Source: CAD feature listing. Evaluate the final solid. Frame: model axes, mm. Give positions to 0.01 mm unless a question says otherwise; leave off trailing zeros. Write each loop counter-clockwise with the first axis right and the second up, starting at its lowest first coordinate (ties: lowest second). Pieces come first, ordered by that corner, then holes. Notation, with made-up numbers: (27, -30) -> (86, -30) arc R36 ccw to (86, 6) -> close; hole circle Ø11 at (-28, 24.25). An arc over 180 degrees is marked (long way). Answer as a JSON object with one key per item and string values. Group by question number.
Item 1: Section query A-A on x = 48. Return the cut outline in (y, z), plus the area to 3 significant figures.
Item 2: Section query D-D on y = -6. Return the cut outline in (x, z).
Item 3: Ray query, probe 1 along Y at (x, z) = (83, 3.1); probe 2 along Y at (x, z) = (78, 2.85); probe 3 along X at (y, z) = (-8, 1.9). Return the intervals inside material, ascending. Write a range as from..to.
Item 4: Section query B-B on y = -23.5. Return the cut outline in (x, z).
Item 5: First-contact query: pin 1 Ø6 at (x, y) = (13, -6) entering from -Z. Flat tip, straight axial feed; report the tip coordinate or a pass-through.
Item 6: Section query C-C on z = 2.85. Return the cut outline in (x, y), plus the area to 3 significant figures.
from build123d import *

# Parameters (mm, degrees)
SKETCH_1_W          = 96
SKETCH_1_H          = 47
EXTRUDE_1_DEPTH     = 6
SKETCH_2_R          = 3.3
CUT_EXTRUDE_1_DEPTH = 10
HOLE_WIZARD_M6_2_D  = 5
FILLET_1_R          = 0.5


with BuildPart() as part:
    # 草图1 → 凸台-拉伸1 (new body)
    with BuildSketch(Plane.XY):
        with Locations((48, -23.5)):
            Rectangle(SKETCH_1_W, SKETCH_1_H)
    extrude(amount=EXTRUDE_1_DEPTH)

    # 草图2 → 切除-拉伸1 (cut)
    with BuildSketch(Plane.XY.offset(6)):
        with Locations((83, -6)):
            Circle(SKETCH_2_R)
        with Locations((83, -41)):
            Circle(SKETCH_2_R)
        with Locations((13, -41)):
            Circle(SKETCH_2_R)
        with Locations((13, -6)):
            Circle(SKETCH_2_R)
    extrude(amount=-CUT_EXTRUDE_1_DEPTH, mode=Mode.SUBTRACT)

    # M6 螺纹孔2 (through all)
    with Locations(Plane.XY.offset(6)):
        with Locations((18, -23.5), (48, -23.5), (78, -23.5)):
            Hole(HOLE_WIZARD_M6_2_D / 2)

    # 圆角1
    fillet_1_edges = [part.edges().sort_by_distance(p)[0] for p in [
        (0, 0, 3),
        (96, 0, 3),
        (96, -47, 3),
        (0, -47, 3),
    ]]
    fillet(fillet_1_edges, radius=FILLET_1_R)


solid = part.part
Worked answers:
{
 "1": {"outline": "(-47, 0) -> (-26, 0) -> (-26, 6) -> (-47, 6) -> close; (-21, 0) -> (0, 0) -> (0, 6) -> (-21, 6) -> close", "area": "252 mm^2"},
 "2": {"outline": "(0, 0) -> (9.7, 0) -> (9.7, 6) -> (0, 6) -> close; (16.3, 0) -> (79.7, 0) -> (79.7, 6) -> (16.3, 6) -> close; (86.3, 0) -> (96, 0) -> (96, 6) -> (86.3, 6) -> close"},
 "3": {"probe 1": "-47..-44.3, -37.7..-9.3, -2.7..0", "probe 2": "-47..-26, -21..0", "probe 3": "0..10.38, 15.62..80.38, 85.62..96"},
 "4": {"outline": "(0, 0) -> (15.5, 0) -> (15.5, 6) -> (0, 6) -> close; (20.5, 0) -> (45.5, 0) -> (45.5, 6) -> (20.5, 6) -> close; (50.5, 0) -> (75.5, 0) -> (75.5, 6) -> (50.5, 6) -> close; (80.5, 0) -> (96, 0) -> (96, 6) -> (80.5, 6) -> close"},
 "5": {"pin 1": "through"},
 "6": {"outline": "(0, -46.5) arc R0.5 ccw to (0.5, -47) -> (95.5, -47) arc R0.5 ccw to (96, -46.5) -> (96, -0.5) arc R0.5 ccw to (95.5, 0) -> (0.5, 0) arc R0.5 ccw to (0, -0.5) -> close; hole circle Ø6.6 at (13, -41); hole circle Ø6.6 at (13, -6); hole circle Ø5 at (18, -23.5); hole circle Ø5 at (48, -23.5); hole circle Ø5 at (78, -23.5); hole circle Ø6.6 at (83, -41); hole circle Ø6.6 at (83, -6)", "area": "4,320 mm^2"}
}
